Autodesk Inventor part; units mm, degrees
ref_plane "YZ Plane" through (0, 0, 0) normal (1, 0, 0) x (0, 1, 0)
ref_plane "XZ Plane" through (0, 0, 0) normal (0, 1, 0) x (-1, 0, 0)
ref_plane "XY Plane" through (0, 0, 0) normal (0, 0, 1) x (1, 0, 0)
sketch "Sketch1" plane through (0, 0, 0) normal (0, 0, 1) x (1, 0, 0)
  line L0 (0, 0) -> (25.4, 0)
  line L1 (25.4, 0) -> (25.4, 25.4)
  line L2 (25.4, 25.4) -> (0, 25.4)
  line L3 (0, 25.4) -> (0, 0)
  line L4 (1.5875, 23.8125) -> (23.8125, 23.8125)
  line L5 (23.8125, 23.8125) -> (23.8125, 1.5875)
  line L6 (23.8125, 1.5875) -> (1.5875, 1.5875)
  line L7 (1.5875, 1.5875) -> (1.5875, 23.8125)
  dimension "d0" = 25.4
  dimension "d1" = 25.4
  dimension "d2" = 1.5875
extrude "Extrusion1" add sketch "Sketch1" against normal blind 914.4
properties part number "1tube_36_frame"
Design review of the part built by this model. Coordinates are the model's own, in mm. A direction names the side the tool comes from. Give positions to 0.01 mm unless a question says otherwise; leave off trailing zeros. Order: outer loops, then holes, each group sorted by start corner. A loop starts at its lowest first (then second) coordinate and runs counter-clockwise, first axis right, second up. Notation, with made-up numbers: (63.25, 19) -> (83.25, 19) arc R9 cw to (83.25, 34) -> close; hole circle Ø2 at (-26, -29). An arc over 180 degrees is marked (long way). Write each question's results on one line, items separated by ' | '. Start each with the question number.
Q1. Machinability: for faces 1 (the flat face through (13, 1.588, -451)), 2 (the flat face through (0, 13, -451)), which of the approach directions +Z, -Z, +X, -X, +Y, -Y give a long, thin tool a straight path to every point of the face, cutting with its end or side? Answer none if there is none.
Q2. For pin 1 (12 mm diameter, centred on x = 11, y = 10, fed in from +Z), flat-tipped, find the tip position at first contact; note if it passes through.
Q3. Mouldability with a two-part tool opening along Y and no side actions: class faces 3 (the flat face through (13, 25.4, -451)), 4 (the flat face through (1.588, 13, -451)), 5 (the flat face through (1, 13, 0)) as +Y half, -Y half, draft (parallel to the pull), parting line (faces both ways), or undercut.
Q4. Wall thickness on L1, parallel to X at y = 4, z = -606: over which ranges is the line inside the solid? List them lowest first. Write a range as from..to.
Q5. Add section C-C on z = -828. Give the boundary of the cut face in (x, y), and give its area (3 significant figures).
Q6. Add section A-A on y = 10. Give the boundary of the cut face in (x, z), and give its area (3 significant figures).
Found:
1) face 1: +Z, -Z | face 2: +Z, -Z, -X, +Y, -Y
2) pin 1: passes through
3) face 3: +Y half | face 4: undercut | face 5: draft
4) L1: x = 0..1.59, 23.81..25.4
5) outline: (0, 0) -> (25.4, 0) -> (25.4, 25.4) -> (0, 25.4) -> close; hole (1.59, 1.59) -> (23.81, 1.59) -> (23.81, 23.81) -> (1.59, 23.81) -> close | area: 151 mm2
6) outline: (0, -914.4) -> (1.59, -914.4) -> (1.59, 0) -> (0, 0) -> close; (23.81, -914.4) -> (25.4, -914.4) -> (25.4, 0) -> (23.81, 0) -> close | area: 2,900 mm2
